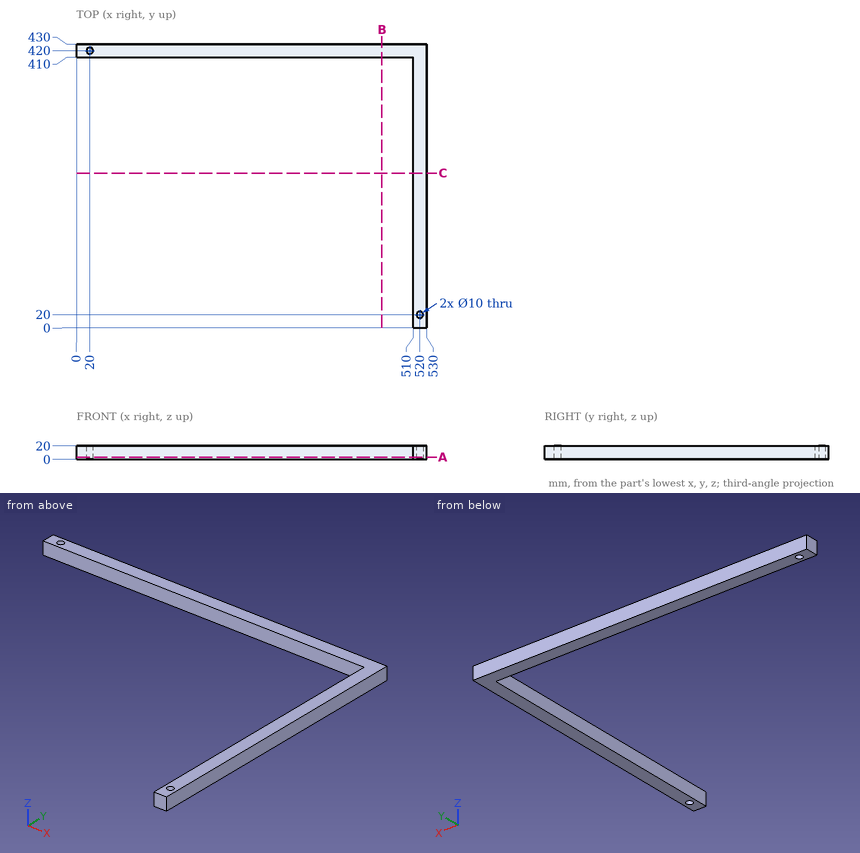
Answer from the drawing. Dimensions are ordinates in mm from the lowest x, y and z of the part. Give positions to 0.01 mm unless a question says otherwise; leave off trailing zeros. Loops run counter-clockwise (first coordinate to the right, second up) from the corner with the lowest first, then second, coordinate; pieces in that order, holes last. Notation, with made-up numbers: (19, 6.25) - (70, 6.25) arc R15 ccw to (70, 25.25) - close; hole circle Ø7 at (71, -37). An arc over 180 degrees is marked (long way). Answer as CSV lines item,"result". Start each with the question number.
Item 1: A cutting plane is placed at B-B on x = 462.5. Determine the outline of the cut face in (y, z), then the cut area to 3 significant figures.
Item 2: A cutting plane is placed at A-A on z = 3. Determine the outline of the cut face in (x, y), then the cut area to 3 significant figures.
Item 3: A cutting plane is placed at C-C on y = 234.5. Determine the outline of the cut face in (x, z), then the cut area to 3 significant figures.
Item 4: Each of these flat-tipped pins is pushed along its axis until it touches: pin 1 (5 mm diameter, centred on y = 127, z = 11, fed in from -X); pin 2 (8 mm diameter, centred on x = 455, z = 2, fed in from -Y). Where does it stop, or does it pass through?
Item 5: Find the intervals of material crossed by line 1 (X direction, y = 420, z = 10.5); line 2 (X direction, y = 20, z = 14); line 3 (Y direction, x = 84, z = 9.25), in increasing order. Write a range as from..to.
Found:
1,outline,"(410, 0) - (430, 0) - (430, 20) - (410, 20) - close"
1,area,"400 mm^2"
2,outline,"(0, 410) - (510, 410) - (510, 0) - (530, 0) - (530, 430) - (0, 430) - close; hole circle Ø10 at (20, 420); hole circle Ø10 at (520, 20)"
2,area,"18,600 mm^2"
3,outline,"(510, 0) - (530, 0) - (530, 20) - (510, 20) - close"
3,area,"400 mm^2"
4,pin 1,"stops at x = 510"
4,pin 2,"stops at y = 410"
5,line 1,"x = 0..15, 25..530"
5,line 2,"x = 510..515, 525..530"
5,line 3,"y = 410..430"
